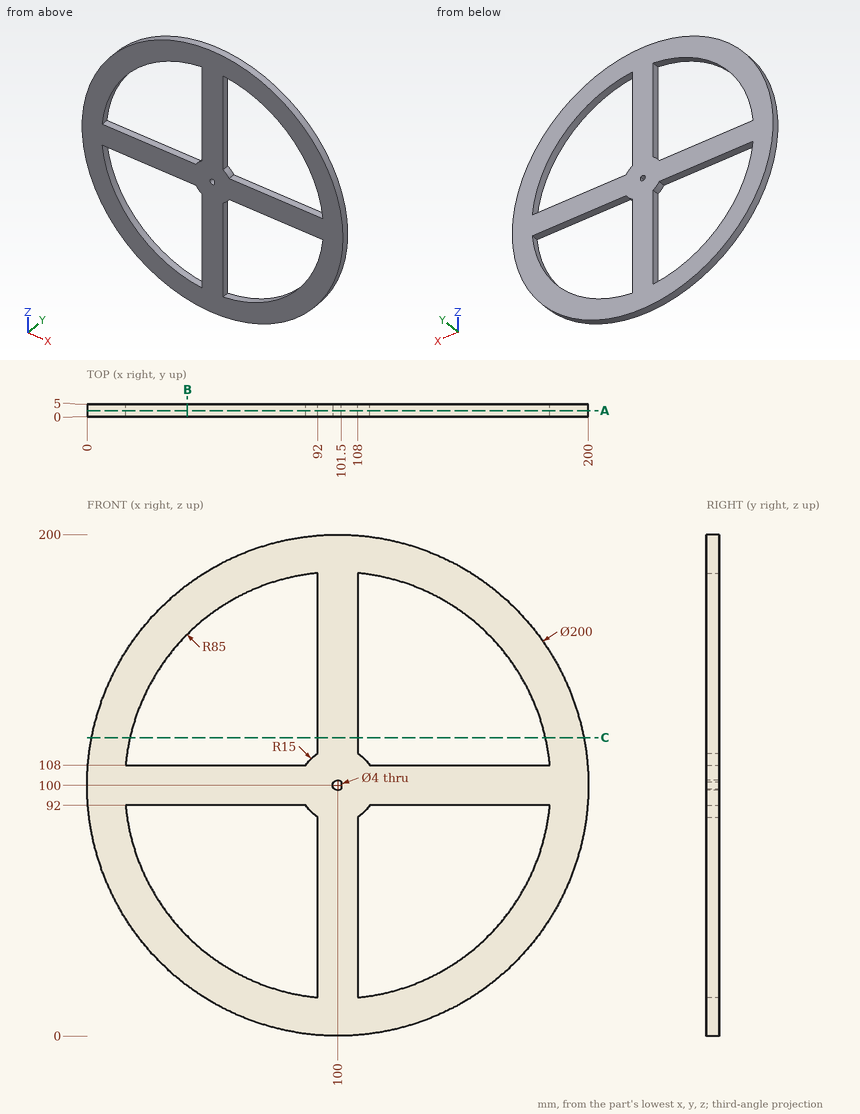
Could you check a few things on this drawing? It's one solid part, dimensions in mm from its lowest x, y, z. Give positions to 0.01 mm unless a question says otherwise; leave off trailing zeros. Write each loop counter-clockwise with the first axis right and the second up, starting at its lowest first coordinate (ties: lowest second). Pieces come first, ordered by that corner, then holes. Notation, with made-up numbers: (84.5, -14) -> (118.5, -14) arc R9 cw to (118.5, -4) -> close; hole circle Ø1 at (-16, -19.5). An arc over 180 degrees is marked (long way). Write item = value, one per line.
(1) I need wall thicknesses on probe 1 along Z at (x, y) = (42, 3.7); probe 2 along Z at (x, y) = (157, 2.7); probe 3 along X at (y, z) = (3.5, 155). Which ranges of each line are inside material? Lowest first, please. Write a range as from..to.
Worked out:
probe_1 = 18.54..37.86, 92..108, 162.14..181.46
probe_2 = 17.84..36.94, 92..108, 163.06..182.16
probe_3 = 16.48..35.19, 92..108, 164.81..183.52
(2) Suppose I cut it at A-A on y = 2.35. Write out the boundary of the cut face in (x, z), then the cut area to 3 significant figures.
Worked out:
outline = circle Ø200 at (100, 100); hole (15.38, 92) arc R85 ccw to (92, 15.38) -> (92, 87.31) arc R15 cw to (87.31, 92) -> close; hole (15.38, 108) -> (87.31, 108) arc R15 cw to (92, 112.69) -> (92, 184.62) arc R85 ccw to start; hole (101.5, 98.68) -> (101.5, 101.32) arc R2 ccw (long way) to start; hole (108, 15.38) arc R85 ccw to (184.62, 92) -> (112.69, 92) arc R15 cw to (108, 87.31) -> close; hole (108, 112.69) arc R15 cw to (112.69, 108) -> (184.62, 108) arc R85 ccw to (108, 184.62) -> close
area = 13,900 mm^2
(3) Suppose I cut it at C-C on z = 119. Write out the boundary of the cut face in (x, y), then the cut area to 3 significant figures.
Worked out:
outline = (1.82, 0) -> (17.15, 0) -> (17.15, 5) -> (1.82, 5) -> close; (92, 0) -> (108, 0) -> (108, 5) -> (92, 5) -> close; (182.85, 0) -> (198.18, 0) -> (198.18, 5) -> (182.85, 5) -> close
area = 233 mm^2
(4) Suppose I cut it at B-B on x = 40. Write out the boundary of the cut face in (y, z).
Worked out:
outline = (0, 20) -> (5, 20) -> (5, 39.79) -> (0, 39.79) -> close; (0, 92) -> (5, 92) -> (5, 108) -> (0, 108) -> close; (0, 160.21) -> (5, 160.21) -> (5, 180) -> (0, 180) -> close
(5) I'm going to push flat-ended pins straight in: P1, Ø3, axis at y = 1, z = 136.5, coming from the -X side (3 decimals); P2, Ø1.5, axis at y = 2.5, z = 54.5, coming from the -X side; P3, Ø1.5, axis at y = 3.5, z = 52.5, coming from the +X side. Where does each tip first touch, or does it pass through?
Worked out:
P1 = 6.325
P2 = 10.57
P3 = 188.4
